Input: part model. Units: mm. Frame: model coordinates. A direction names the side the tool comes from. Coordinates: 2 decimals unless noted, no trailing zeros. Loops run counter-clockwise (first coordinate to the right, second up) from the corner with the lowest first, then second, coordinate; pieces in that order, holes last.
```python
from build123d import *

# Parameters (mm, degrees)
F0_R     = 1.5
F1_DEPTH = 7
F2_DEPTH = 7
F3_R     = 22
F4_DEPTH = 5.5


with BuildPart() as f1:
    # F0 (on Top) → F1 (new body)
    with BuildSketch(Plane.XY):
        with BuildLine():
            ThreePointArc((-26.6379310345, -4.4068844099), (-27, 0), (-26.6379310345, 4.4068844099))
            ThreePointArc((-26.6379310345, 4.4068844099), (-34, 0), (-26.6379310345, -4.4068844099))
        make_face()
        with Locations((-29, 0)):
            Circle(F0_R, mode=Mode.SUBTRACT)
    extrude(amount=F1_DEPTH)



with BuildPart() as f1b:
    # F0 (on Top) → F1, piece 2 (new body)
    with BuildSketch(Plane.XY):
        with BuildLine():
            ThreePointArc((26.6379310345, 4.4068844099), (26.9093305187, 2.21086658), (27, 0))
            ThreePointArc((27, 0), (26.9093305187, -2.21086658), (26.6379310345, -4.4068844099))
            ThreePointArc((26.6379310345, -4.4068844099), (31.5680396388, -4.2901249881), (34, 0))
            ThreePointArc((34, 0), (31.5680396388, 4.2901249881), (26.6379310345, 4.4068844099))
        make_face()
        with Locations((29, 0)):
            Circle(F0_R, mode=Mode.SUBTRACT)
    extrude(amount=F1_DEPTH)


with BuildPart() as f1_1:
    add(f1.part)

    add(f1b.part)  # F2 merges F1b
    # F0 (on Top) → F2 (join)
    with BuildSketch(Plane.XY):
        with BuildLine():
            ThreePointArc((-24, 0), (-24.7098750119, 2.5680396388), (-26.6379310345, 4.4068844099))
            ThreePointArc((-26.6379310345, 4.4068844099), (-27, 0), (-26.6379310345, -4.4068844099))
            ThreePointArc((-26.6379310345, -4.4068844099), (-24.7098750119, -2.5680396388), (-24, 0))
        make_face()
        with BuildLine():
            ThreePointArc((26.6379310345, -4.4068844099), (26.9093305187, -2.21086658), (27, 0))
            ThreePointArc((27, 0), (26.9093305187, 2.21086658), (26.6379310345, 4.4068844099))
            ThreePointArc((26.6379310345, 4.4068844099), (24, 0), (26.6379310345, -4.4068844099))
        make_face()
        with BuildLine():
            ThreePointArc((26.6379310345, -4.4068844099), (24, 0), (26.6379310345, 4.4068844099))
            ThreePointArc((26.6379310345, 4.4068844099), (0, 27), (-26.6379310345, 4.4068844099))
            ThreePointArc((-26.6379310345, 4.4068844099), (-24.7098750119, 2.5680396388), (-24, 0))
            ThreePointArc((-24, 0), (-24.7098750119, -2.5680396388), (-26.6379310345, -4.4068844099))
            ThreePointArc((-26.6379310345, -4.4068844099), (0, -27), (26.6379310345, -4.4068844099))
        make_face()
    extrude(amount=F2_DEPTH)

    # F3 (on face) → F4 (cut)
    with BuildSketch(Plane.XY.offset(7)):
        Circle(F3_R)
    extrude(amount=-F4_DEPTH, mode=Mode.SUBTRACT)


solid = f1_1.part
```
Item 1: Line query: L1, parallel to Y at x = 29, z = 4.75; L2, parallel to Z at x = 5.5, y = 19.5; L3, parallel to X at y = -10, z = 2. Output: solid intervals per line, ascending.
Result:
L1: y = -5 to -1.5, 1.5 to 5
L2: z = 0 to 1.5
L3: x = -25.08 to -19.6, 19.6 to 25.08
Item 2: Section query D-D (y = 17). Output: boundary loops of the cut face in (x, z), then the cut area to 3 significant figures.
Result:
outline: (-20.98, 0) - (20.98, 0) - (20.98, 7) - (13.96, 7) - (13.96, 1.5) - (-13.96, 1.5) - (-13.96, 7) - (-20.98, 7) - close
area: 140 mm2
Item 3: Section query A-A (x = -29). Output: boundary loops of the cut face in (y, z).
Result:
outline: (-5, 0) - (-1.5, 0) - (-1.5, 7) - (-5, 7) - close; (1.5, 0) - (5, 0) - (5, 7) - (1.5, 7) - close
Item 4: Mould query, pull axis X, two halves, no side actions, for faces 3 (the face through (2.4, 22.1, 7)), 4 (the face through (0, 0, 1.5)). Classes: +X half, -X half, draft (parallel to the pull), parting line (faces both ways), or undercut.
Result:
face 3: draft
face 4: undercut
Item 5: Contact query for a flat-ended pin moving along its axis: P1, Ø1.8, axis at x = -29, y = 0, coming from the +Z side. Output: stop coordinate, or through.
Result:
P1: passes through
Item 6: Section query C-C (x = 0). Output: boundary loops of the cut face in (y, z), then the cut area to 3 significant figures.
Result:
outline: (-27, 0) - (27, 0) - (27, 7) - (22, 7) - (22, 1.5) - (-22, 1.5) - (-22, 7) - (-27, 7) - close
area: 136 mm2
Item 7: Section query B-B (z = 4.5). Output: boundary loops of the cut face in (x, y), then the cut area to 3 significant figures.
Result:
outline: (-26.64, -4.41) arc R27 ccw to (26.64, -4.41) arc R5 ccw (long way) to (26.64, 4.41) arc R27 ccw to (-26.64, 4.41) arc R5 ccw (long way) to start; hole circle Ø3 at (-29, 0); hole circle Ø44 at (0, 0); hole circle Ø3 at (29, 0)
area: 875 mm2
Item 8: Reachability of faces 1 (the face through (27.5, 0.07, 3.45)), 2 (the face through (-4.769, -21.477, 4.288)) from +Z, -Z, +X, -X, +Y, -Y: full face, straight path, thin tool, end or side. Return the list, or none.
Result:
face 1: +Z, -Z
face 2: +Z
